Here's how the part is built. I have some questions about the finished solid (model axes, mm). Face numbers are marked on the shaded views. A direction names the side the tool comes from. Give positions to 0.01 mm unless a question says otherwise; leave off trailing zeros. Loops run counter-clockwise (first coordinate to the right, second up) from the corner with the lowest first, then second, coordinate; pieces in that order, holes last. Notation, with made-up numbers: M 54.25,4 L 110.25,4 A24 ccw 110.25,37 Z; hole C -35.5,27 d8. An arc over 180 degrees is marked long. Answer as CSV lines item,"result". Start each with the question number.
Item 1: Will these pins go through, and if not, where does the flat tip stop? P1, Ø3, axis at y = 51, z = 11.5, coming from the +X side; P2, Ø0.7, axis at x = 4.5, y = 50.5, coming from the +Z side; P3, Ø6, axis at y = -35.5, z = 12.5, coming from the +X side.
Item 2: If we mould it in two halves opening along X, with no side actions, what happens to the marked faces 3 and 4? For each: released by +X, released by -X, zero draft, split by the parting line, or undercut.
Item 3: I want a section at C-C on x = -37.5. List the corners of the cut face in (y, z) for me, plus the area to 3 significant figures.
Item 4: I want a section at A-A on y = 35.5. List the corners of the cut face in (x, z) for me, plus the area to 3 significant figures.
Item 5: I want a section at D-D on y = 0. List the corners of the cut face in (x, z) for me.
Item 6: If I drill on line 1 along Y through (x, z) = (-25, 5.5); line 2 along X through (y, z) = (-42.5, 5.75); line 3 along X through (y, z) = (42.5, 5), over which ranges is the centre line in solid material (lowest first)? Write a range as from..to.
Item 7: For the marked faces 1 and 2, which set-ups out of +Z, -Z, +X, -X, +Y, -Y let a thin tool reach every point of the face, with its end or its side?
Item 8: I want a section at B-B on x = 20. Give the number of separate pieces and of enclosed holes in the cut face, plus the area to 3 significant figures.
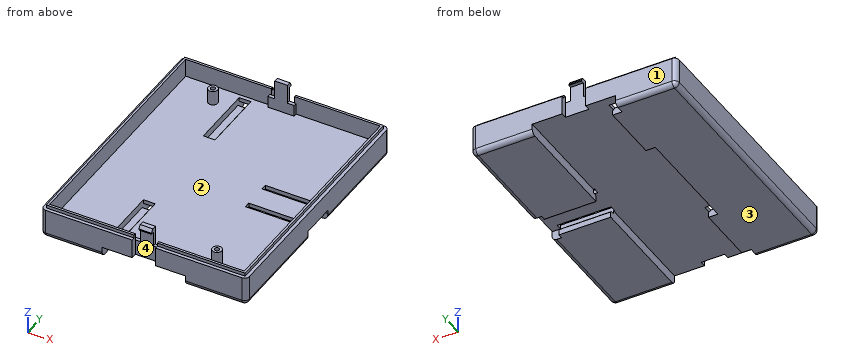
from build123d import *

# Parameters (mm, degrees)
PAD002_DEPTH    = 53.5
SKETCH009_W     = 83
SKETCH009_H     = 102.2
POCKET005_DEPTH = 7.9
SKETCH010_R     = 2
SKETCH010_R_2   = 1
PAD003_DEPTH    = 6.2
SKETCH011_W     = 3
SKETCH011_H     = 25
PAD004_DEPTH    = 4
CHAMFER001_SIZE = 1
POCKET006_DEPTH = 26.1
CHAMFER002_SIZE = 0.5
SKETCH013_W     = 4.3
SKETCH013_H     = 15
POCKET007_DEPTH = 4
SKETCH014_W     = 23.1
SKETCH014_H     = 2.5
SKETCH014_W_2   = 5
SKETCH014_H_2   = 27
POCKET008_DEPTH = 1.7
SKETCH015_W     = 3.85
SKETCH015_H     = 13.9
POCKET009_DEPTH = 5
PAD005_DEPTH    = 2.7
SKETCH017_W     = 1.45
SKETCH017_H     = 6.7
PAD006_DEPTH    = 5.6
FILLET002_R     = 2
SKETCH018_W     = 87.7
SKETCH018_H     = 107
SKETCH018_W_2   = 84.84
SKETCH018_H_2   = 104.14
POCKET010_DEPTH = 1.4


with BuildPart() as part:
    # Sketch008 → Pad002 (new body, symmetric)
    with BuildSketch(Plane.XZ):
        Polygon((43.85, 9.6), (-43.85, 9.6), (-43.85, -4.3), (-17.75, -4.3), (-17.75, 0), (17.75, 0), (17.75, -4.3), (43.85, -4.3), align=None)
    extrude(amount=PAD002_DEPTH, both=True)

    # Sketch009 (on Face1 of Pad002) → Pocket005 (cut)
    with BuildSketch(Plane(origin=(0, 0, 9.6), x_dir=(-1, 0, 0), z_dir=(0, 0, 1))):
        Rectangle(SKETCH009_W, SKETCH009_H)
    extrude(amount=-POCKET005_DEPTH, mode=Mode.SUBTRACT)

    # Sketch010 (on Face15 of Pocket005) → Pad003 (join)
    with BuildSketch(Plane(origin=(0, 0, 1.7), x_dir=(-1, 0, 0), z_dir=(0, 0, 1))):
        with Locations((25, -42.5)):
            Circle(SKETCH010_R)
        with Locations((25, -42.5)):
            Circle(SKETCH010_R_2, mode=Mode.SUBTRACT)
        with Locations((-25, 42.5)):
            Circle(SKETCH010_R)
        with Locations((-25, 42.5)):
            Circle(SKETCH010_R_2, mode=Mode.SUBTRACT)
    extrude(amount=PAD003_DEPTH)

    # Sketch011 (on Face12 of Pad003) → Pad004 (join)
    with BuildSketch(Plane(origin=(-17.75, 0, 0), x_dir=(0, 0, 1), z_dir=(1, 0, 0))):
        with Locations((-2.8, -36)):
            Rectangle(SKETCH011_W, SKETCH011_H)
        with Locations((-2.8, 36)):
            Rectangle(SKETCH011_W, SKETCH011_H)
    extrude(amount=PAD004_DEPTH)

    # Chamfer001
    chamfer001_edges = [part.edges().sort_by_distance(p)[0] for p in [
        (-13.75, 36, -1.3),
        (-13.75, -36, -1.3),
    ]]
    chamfer(chamfer001_edges, length=CHAMFER001_SIZE)

    # Sketch012 (on Face19 of Chamfer001) → Pocket006 (cut)
    with BuildSketch(Plane(origin=(43.85, 0, 0), x_dir=(0, 0, 1), z_dir=(1, 0, 0))):
        Polygon((0, 7.5), (-1.4, 7.5), (-1.4, 5.5), (-6.4, 5.5), (-6.4, -5.5), (-1.4, -5.5), (-1.4, -7.500011), (0, -7.5), align=None)
    extrude(amount=-POCKET006_DEPTH, mode=Mode.SUBTRACT)

    # Chamfer002
    chamfer002_edges = [part.edges().sort_by_distance(p)[0] for p in [
        (30.8, -5.5, -1.4),
        (30.8, 5.5, -1.4),
    ]]
    chamfer(chamfer002_edges, length=CHAMFER002_SIZE)

    # Sketch013 (on Face9 of Chamfer002) → Pocket007 (cut)
    with BuildSketch(Plane(origin=(43.85, 0, 0), x_dir=(0, 0, 1), z_dir=(1, 0, 0))):
        with Locations((-2.15, 0)):
            Rectangle(SKETCH013_W, SKETCH013_H)
    extrude(amount=-POCKET007_DEPTH, mode=Mode.SUBTRACT)

    # Sketch014 (on Face33 of Pocket007) → Pocket008 (cut)
    with BuildSketch(Plane(origin=(0, 0, 1.7), x_dir=(-1, 0, 0), z_dir=(0, 0, 1))):
        with Locations((-28.8, -6.25)):
            Rectangle(SKETCH014_W, SKETCH014_H)
        with Locations((15.25, -36)):
            Rectangle(SKETCH014_W_2, SKETCH014_H_2)
        with Locations((-28.8, 6.25)):
            Rectangle(SKETCH014_W, SKETCH014_H)
        with Locations((15.25, 36)):
            Rectangle(SKETCH014_W_2, SKETCH014_H_2)
    extrude(amount=-POCKET008_DEPTH, mode=Mode.SUBTRACT)

    # Sketch015 → Pocket009 (cut, symmetric)
    with BuildSketch(Plane.YZ):
        with Locations((51.575, 2.65)):
            Rectangle(SKETCH015_W, SKETCH015_H)
    pocket009 = extrude(amount=POCKET009_DEPTH, both=True, mode=Mode.SUBTRACT)

    # Sketch016 → Pad005 (join, symmetric)
    with BuildSketch(Plane.YZ):
        Polygon((49.65, 0), (49.65, 15), (51.5, 15), (52.5, 13.6), (52.5, 13.1), (51.1, 13.1), (51.1, 0), align=None)
    pad005 = extrude(amount=PAD005_DEPTH, both=True)

    # Sketch017 → Pad006 (join, symmetric)
    with BuildSketch(Plane.YZ):
        with Locations((50.375, 3.35)):
            Rectangle(SKETCH017_W, SKETCH017_H)
    pad006 = extrude(amount=PAD006_DEPTH, both=True)

    # Mirrored003: Pocket009, Pad005, Pad006 across XZ
    add(pocket009.mirror(Plane.XZ), mode=Mode.SUBTRACT)
    add(pad005.mirror(Plane.XZ))
    add(pad006.mirror(Plane.XZ))

    # Fillet002
    fillet002_edges = [part.edges().sort_by_distance(p)[0] for p in [
        (43.85, 53.5, 2.65),
        (43.85, 30.5, -4.3),
        (30.8, 53.5, -4.3),
        (-30.8, 53.5, -4.3),
        (-43.85, 53.5, 2.65),
        (43.85, -30.5, -4.3),
        (43.85, -53.5, 2.65),
        (30.8, -53.5, -4.3),
        (-30.8, -53.5, -4.3),
        (-43.85, -53.5, 2.65),
        (-43.85, 0, -4.3),
    ]]
    fillet(fillet002_edges, radius=FILLET002_R)

    # Sketch018 (on Face71 of Fillet002) → Pocket010 (cut)
    with BuildSketch(Plane(origin=(0, 0, 9.6), x_dir=(-1, 0, 0), z_dir=(0, 0, 1))):
        Rectangle(SKETCH018_W, SKETCH018_H)
        Rectangle(SKETCH018_W_2, SKETCH018_H_2, mode=Mode.SUBTRACT)
    extrude(amount=-POCKET010_DEPTH, mode=Mode.SUBTRACT)


solid = part.part
Result:
1,P1,"x = 2.7"
1,P2,"z = 6.7"
1,P3,"x = 42.42"
2,face 3,"zero draft"
2,face 4,"undercut"
3,outline,"M -53.5,-2.3 A2 ccw -51.5,-4.3 L 51.5,-4.3 A2 ccw 53.5,-2.3 L 53.5,8.2 L 52.07,8.2 L 52.07,9.6 L 51.1,9.6 L 51.1,1.7 L -51.1,1.7 L -51.1,9.6 L -52.07,9.6 L -52.07,8.2 L -53.5,8.2 Z"
3,area,"674 mm^2"
4,outline,"M -43.85,-2.3 A2 ccw -41.85,-4.3 L -13.75,-4.3 L -13.75,-2.3 L -14.75,-1.3 L -17.75,-1.3 L -17.75,1.7 L -41.5,1.7 L -41.5,9.6 L -42.42,9.6 L -42.42,8.2 L -43.85,8.2 Z; M -12.75,0 L 17.75,0 L 17.75,-4.3 L 41.85,-4.3 A2 ccw 43.85,-2.3 L 43.85,8.2 L 42.42,8.2 L 42.42,9.6 L 41.5,9.6 L 41.5,1.7 L -12.75,1.7 Z"
4,area,"408 mm^2"
5,outline,"M -43.85,-2.3 A2 ccw -41.85,-4.3 L -17.75,-4.3 L -17.75,0 L 43.85,0 L 43.85,8.2 L 42.42,8.2 L 42.42,9.6 L 41.5,9.6 L 41.5,1.7 L -41.5,1.7 L -41.5,9.6 L -42.42,9.6 L -42.42,8.2 L -43.85,8.2 Z"
6,line 1,"-53.5..-51.1, 40.5..41.5, 43.5..44.5, 51.1..53.5"
6,line 2,"-43.85..-41.5, 23..24, 26..27, 41.5..43.85"
6,line 3,"-43.85..-41.5, -27..-26, -24..-23, 41.5..43.85"
7,face 1,"+Z, -Z, +X, -X, +Y"
7,face 2,"+Z"
8,separate pieces,"3"
8,enclosed holes,"0"
8,area,"613 mm^2"
